from build123d import *

# Parameters (mm, degrees)
SKETCH_1_R      = 10
EXTRUDE_1_DEPTH = 30
SKETCH_2_R      = 13
EXTRUDE_2_DEPTH = 5
EXTRUDE_3_DEPTH = 4
SKETCH_5_R      = 6
EXTRUDE_4_DEPTH = 10


with BuildPart() as part:
    # 草图1 → 拉伸1 (new body)
    with BuildSketch(Plane.XY):
        Circle(SKETCH_1_R)
    extrude_1 = extrude(amount=-EXTRUDE_1_DEPTH)

    # 草图2 → 拉伸2 (add)
    with BuildSketch(Plane(origin=(0, 0, -30), x_dir=(-1, 0, 0), z_dir=(0, 0, -1))):
        Circle(SKETCH_2_R)
    extrude_2 = extrude(amount=EXTRUDE_2_DEPTH)

    # 草图3 → 拉伸3 (add)
    with BuildSketch(Plane(origin=(0, 0, -35), x_dir=(-1, 0, 0), z_dir=(0, 0, -1))):
        with BuildLine():
            Line((-9.2, 13.62938003), (23.971428571, 21.41759719))
            ThreePointArc((23.971428571, 21.41759719), (51, 0), (23.971428571, -21.41759719))
            Line((23.971428571, -21.41759719), (-9.2, -13.62938003))
            ThreePointArc((-9.2, -13.62938003), (-20, 0), (-9.2, 13.62938003))
        make_face()
    extrude_3 = extrude(amount=EXTRUDE_3_DEPTH)

    # 草图5 → 拉伸4 (add)
    with BuildSketch(Plane(origin=(0, 0, -39), x_dir=(-1, 0, 0), z_dir=(0, 0, -1))):
        with Locations((34.589570742, 0)):
            Circle(SKETCH_5_R)
    extrude_4 = extrude(amount=EXTRUDE_4_DEPTH)

    # 镜向2: 拉伸1, 拉伸2, 拉伸3, 拉伸4 across plane
    add(extrude_1.mirror(Plane(origin=(-34.589570742, 0, -49), x_dir=(1, 0, 0), z_dir=(0, 0, -1))))
    add(extrude_2.mirror(Plane(origin=(-34.589570742, 0, -49), x_dir=(1, 0, 0), z_dir=(0, 0, -1))))
    add(extrude_3.mirror(Plane(origin=(-34.589570742, 0, -49), x_dir=(1, 0, 0), z_dir=(0, 0, -1))))
    add(extrude_4.mirror(Plane(origin=(-34.589570742, 0, -49), x_dir=(1, 0, 0), z_dir=(0, 0, -1))))


solid = part.part
The listing builds one solid part. Answer for the finished solid, in the listing's coordinates (mm). A direction names the side the tool comes from. Round coordinates to 2 decimals unless told otherwise and drop trailing zeros. Write each loop counter-clockwise with the first axis right and the second up, starting at its lowest first coordinate (ties: lowest second). Pieces come first, ordered by that corner, then holes. Notation, with made-up numbers: M 9,10 L 50,10 A23 cw 50,37 Z; hole C 63,1.5 d2. An arc over 180 degrees is marked long. Write each question's results on one line, items separated by ' | '. Start each with the question number.
Item 1: Find section A-A on y = 0. Write down the section's boundary in (x, z), and give its area (3 significant figures).
Item 2: Which of the six approach directions +Z, -Z, +X, -X, +Y, -Y give full straight-line access (tool end or side, diameter ignored) to faces 4 (the cylindrical face through (-2.17, -9.76, -14.79)), 5 (the cylindrical face through (20, 0, -61)), 6 (the cylindrical face through (10.316, -7.91, -65.535))?
Item 3: Find section B-B on x = -45.5. Write down the section's boundary in (y, z), and give its area (3 significant figures).
Item 4: Find section C-C on z = -9. Write down the section's boundary in (x, y), and give its area (3 significant figures).
Item 5: Find section D-D on x = -4. Write down the section's boundary in (y, z).
Item 6: Given pin 1 Ø22 at (x, y) = (-33, 11) entering from -Z; pin 2 Ø10 at (x, z) = (-27.5, -69) entering from -Y; pin 3 Ø10 at (y, z) = (3, -63.5) entering from -X; pin 4 Ø1.5 at (y, z) = (-1.5, -29.5) entering from +X, each flat-ended and moving along its own axis, determine where each tip first touches the part or whether it passes through.
Item 7: Straight lines are drawn through the part: probe 1 along Z at (x, y) = (-30, 7); probe 2 along Z at (x, y) = (9.5, 5); probe 3 along Z at (x, y) = (-34.5, -2). For each, find the intervals that lie inside material, in ascending order.
Item 8: The mould has two halves that part along Z. Classify faces 1 (the cylindrical face through (10.316, -7.91, -32.465)), 2 (the flat face through (-7, -8, -30)), 3 (the flat face through (-16, 0, -39)): +Z half, -Z half, draft (parallel to the pull), parting line (faces both ways), or undercut.
Answer block:
1) outline: M -51,-63 L -13,-63 L -13,-68 L -10,-68 L -10,-98 L 10,-98 L 10,-68 L 13,-68 L 13,-63 L 20,-63 L 20,-59 L -28.59,-59 L -28.59,-39 L 20,-39 L 20,-35 L 13,-35 L 13,-30 L 10,-30 L 10,0 L -10,0 L -10,-30 L -13,-30 L -13,-35 L -51,-35 L -51,-39 L -40.59,-39 L -40.59,-59 L -51,-59 Z | area: 2,270 mm²
2) face 4: +Z | face 5: +Z, -Z, +X | face 6: -Z
3) outline: M -14.55,-63 L 14.55,-63 L 14.55,-59 L -14.55,-59 Z; M -14.55,-39 L 14.55,-39 L 14.55,-35 L -14.55,-35 Z | area: 233 mm²
4) outline: C 0,0 d20 | area: 314 mm²
5) outline: M -16.73,-63 L -12.37,-63 L -12.37,-68 L -9.17,-68 L -9.17,-98 L 9.17,-98 L 9.17,-68 L 12.37,-68 L 12.37,-63 L 16.73,-63 L 16.73,-59 L -16.73,-59 Z; M -16.73,-39 L 16.73,-39 L 16.73,-35 L 12.37,-35 L 12.37,-30 L 9.17,-30 L 9.17,0 L -9.17,0 L -9.17,-30 L -12.37,-30 L -12.37,-35 L -16.73,-35 Z
6) pin 1: stops at z = -63 | pin 2: passes through | pin 3: stops at x = -51 | pin 4: stops at x = 12.97
7) probe 1: z = -63 to -59, -39 to -35 | probe 2: z = -68 to -59, -39 to -30 | probe 3: z = -63 to -35
8) face 1: draft | face 2: +Z half | face 3: undercut
